Source: CAD feature listing. Evaluate the final solid. Frame: model axes, mm. Round coordinates to 2 decimals unless told otherwise and drop trailing zeros. Order: outer loops, then holes, each group sorted by start corner. A loop starts at its lowest first (then second) coordinate and runs counter-clockwise, first axis right, second up. Notation, with made-up numbers: (32, 41) - (80, 41) arc R11 cw to (80, 46) - close; hole circle Ø1 at (-10.5, 89). An arc over 180 degrees is marked (long way). Return JSON: item names as keys, results as strings. Group by question number.
1) Section D-D, the plane y = 4.5. Give the number of separate pieces and of enclosed holes in the cut face, plus the area to 3 significant figures.
2) Section C-C, the plane y = -3. Return loops of the section in (x, z), plus the area to 3 significant figures.
3) Contact query for a flat-ended pin moving along its axis: P1, Ø3, axis at x = -18.1, y = 3.97, coming from the +Z side. Output: stop coordinate, or through.
4) Ray query, line 1 (Y direction, x = -14.5, z = 0.5); line 2 (X direction, y = 6.5, z = 0.8); line 3 (X direction, y = 4.25, z = 0.65). Return the intervals inside material, ascending. Write a range as from..to.
5) Section A-A, the plane y = 6.5. Return loops of the section in (x, z).
6) Section B-B, the plane x = -1. Return loops of the section in (y, z).
7) Mould query, pull axis X, two halves, no side actions, for faces 1 (the flat face through (-18.079, -3.318, 0.704)), 2 (the cylindrical face through (8.047, 3.919, 0.704)), 3 (the flat face through (-3, 11, 1.4)). Classes: pulls with the +X half, pulls with the -X half, needs draft (parallel to the pull), parting line crosses it, or undercut.
```python
from build123d import *

# Parameters (mm, degrees)
SKETCH4_R           = 1.2500000000000009
SKETCH4_R_2         = 1.2499999999999993
BOSS_EXTRUDE1_DEPTH = 1.4
CHAMFER1_SIZE       = 0.4


with BuildPart() as part:
    # Sketch4 → Boss-Extrude1 (new body)
    # profile 1 of 8: a face of its own
    with BuildSketch(Plane(origin=(-1.7e-16, 0, 1.4000000000000032), x_dir=(-1, 0, -1.2e-16), z_dir=(1.2e-16, 0, -1))):
        Polygon((-7.546190091207485, 10.174212835332735), (-7.046190091207492, 10.174212835332735), (15.853809908792503, 10.174212835332744), (16.35380990879248, 10.174212835332744), (16.35380990879248, 10.674212835332737), (-7.546190091207485, 10.674212835332732), align=None)
    # profile 2 of 8: a face of its own
    with BuildSketch(Plane(origin=(-1.7e-16, 0, 1.4000000000000032), x_dir=(-1, 0, -1.2e-16), z_dir=(1.2e-16, 0, -1))):
        Polygon((-11.686815091207489, 10.17421283533274), (-7.546190091207485, 10.174212835332735), (-7.546190091207485, 10.674212835332732), (16.35380990879248, 10.674212835332737), (16.35380990879248, 10.174212835332744), (20.7538099087925, 10.17421283533274), (15.853809908792503, 12.174212835332744), (-7.046190091207496, 12.174212835332744), (-11.65105221022055, 10.294677276551901), align=None)
    # profile 3 of 8: a face of its own
    with BuildSketch(Plane(origin=(-1.7e-16, 0, 1.4000000000000032), x_dir=(-1, 0, -1.2e-16), z_dir=(1.2e-16, 0, -1))):
        with BuildLine():
            Line((16.35380990879248, 10.174212835332744), (16.353809908792496, -2.225787164667265))
            Line((16.353809908792496, -2.225787164667266), (20.4739831765189, -2.2257871646672647))
            ThreePointArc((20.473983176518885, -2.2257871646672385), (20.614466316717532, -2.0161736201746514), (20.753809908793457, -1.8058008223556463))
            Line((20.753809908792505, -1.805800822355394), (20.7538099087925, 10.17421283533274))
            Line((20.7538099087925, 10.17421283533274), (16.35380990879248, 10.174212835332744))
        make_face()
        with Locations(Location((18.103809908792506, 3.9742128353327333, 0), (0, 0, 180))):
            Circle(SKETCH4_R, mode=Mode.SUBTRACT)
    # profile 4 of 8: a face of its own
    with BuildSketch(Plane(origin=(-1.7e-16, 0, 1.4000000000000032), x_dir=(-1, 0, -1.2e-16), z_dir=(1.2e-16, 0, -1))):
        with BuildLine():
            Line((-7.54619009120748, -2.7257871646672593), (-7.54619009120748, -2.225787164667266))
            Line((-7.54619009120748, -2.225787164667266), (-11.946190091207495, -2.225787164667265))
            Line((-11.946190091207495, -2.225787164667265), (-7.046190091207487, -4.225787164667266))
            Line((-7.046190091207487, -4.225787164667266), (15.853809908792512, -4.225787164667266))
            Line((15.85380990879251, -4.225787164667266), (20.36710720596046, -2.383625002557896))
            ThreePointArc((20.367107205960004, -2.3836250025573023), (20.420626069676963, -2.3047608484368673), (20.473983176518885, -2.2257871646672385))
            Line((20.4739831765189, -2.2257871646672647), (16.353809908792496, -2.225787164667266))
            Line((16.353809908792496, -2.225787164667265), (16.353809908792496, -2.7257871646672562))
            Line((16.353809908792496, -2.725787164667256), (-7.546190091207482, -2.7257871646672593))
        make_face()
    # profile 5 of 8: a face of its own
    with BuildSketch(Plane(origin=(-1.7e-16, 0, 1.4000000000000032), x_dir=(-1, 0, -1.2e-16), z_dir=(1.2e-16, 0, -1))):
        Polygon((15.853809908792512, -2.225787164667266), (-7.046190091207487, -2.225787164667266), (-7.54619009120748, -2.225787164667266), (-7.54619009120748, -2.7257871646672593), (16.353809908792496, -2.725787164667256), (16.353809908792496, -2.225787164667265), align=None)
    # profile 6 of 8: a face of its own
    with BuildSketch(Plane(origin=(-1.7e-16, 0, 1.4000000000000032), x_dir=(-1, 0, -1.2e-16), z_dir=(1.2e-16, 0, -1))):
        Polygon((-11.946190091207495, -2.225787164667265), (-7.54619009120748, -2.225787164667266), (-7.546190091207485, 10.174212835332735), (-11.686815091207489, 10.17421283533274), (-11.946190091207496, 9.300528624806402), align=None)
        with Locations(Location((-9.296190091207496, 3.9742128353327333, 0), (0, 0, 180))):
            Circle(SKETCH4_R_2, mode=Mode.SUBTRACT)
    # profile 7 of 8: a face of its own
    with BuildSketch(Plane(origin=(-1.7e-16, 0, 1.4000000000000032), x_dir=(-1, 0, -1.2e-16), z_dir=(1.2e-16, 0, -1))):
        Polygon((15.853809908792503, 10.174212835332742), (15.85380990879251, -2.225787164667266), (16.353809908792496, -2.225787164667266), (16.35380990879248, 10.174212835332744), align=None)
    # profile 8 of 8: a face of its own
    with BuildSketch(Plane(origin=(-1.7e-16, 0, 1.4000000000000032), x_dir=(-1, 0, -1.2e-16), z_dir=(1.2e-16, 0, -1))):
        Polygon((-7.54619009120748, -2.225787164667266), (-7.046190091207487, -2.225787164667266), (-7.046190091207492, 10.174212835332735), (-7.546190091207485, 10.174212835332735), align=None)
    extrude(amount=BOSS_EXTRUDE1_DEPTH)

    # Chamfer1
    chamfer1_edges = [part.edges().sort_by_distance(p)[0] for p in [
        (8.046190091207496, 3.974212835332733, 1.4000000000000041),
        (-19.353809908792506, 3.974212835332733, 1.4000000000000008),
        (-4.403809908792507, 10.17421283533274, 1.4000000000000028),
        (7.04619009120749, 3.974212835332734, 1.4000000000000041),
        (-4.403809908792514, -2.2257871646672656, 1.4000000000000028),
        (-15.853809908792506, 3.9742128353327377, 1.4000000000000012),
        (11.798621150714023, 9.797602950679153, 1.4000000000000048),
        (9.348621150714022, 11.234445055942324, 1.4000000000000044),
        (-4.403809908792503, 12.174212835332744, 1.4000000000000028),
        (-18.303809908792502, 11.174212835332742, 1.400000000000001),
        (-20.753809908792505, 4.184206006488673, 1.4000000000000008),
        (-20.56153855062731, -2.095435686482624, 1.4000000000000008),
        (-18.110458557376482, -3.3047060836125812, 1.400000000000001),
        (-4.403809908792512, -4.225787164667266, 1.4000000000000028),
        (9.496190091207492, -3.2257871646672656, 1.4000000000000044),
        (11.946190091207495, 3.5373707300695685, 1.4000000000000048),
        (11.798621150714023, 9.797602950679153, 4.78e-15),
        (7.04619009120749, 3.974212835332734, 4.19e-15),
        (-4.40380990879251, -2.2257871646672656, 2.79e-15),
        (-15.853809908792506, 3.9742128353327377, 1.39e-15),
        (8.046190091207496, 3.974212835332733, 4.32e-15),
        (-19.353809908792506, 3.974212835332733, 9.6e-16),
        (9.348621150714022, 11.234445055942324, 4.48e-15),
        (-4.403809908792503, 12.174212835332744, 2.79e-15),
        (-18.303809908792502, 11.174212835332742, 1.09e-15),
        (-20.753809908792505, 4.184206006488673, 7.9e-16),
        (-20.56153855062727, -2.095435686482599, 8.1e-16),
        (-18.110458557376482, -3.3047060836125812, 1.11e-15),
        (-4.403809908792512, -4.225787164667266, 2.79e-15),
        (9.496190091207492, -3.2257871646672656, 4.49e-15),
        (11.946190091207495, 3.5373707300695685, 4.79e-15),
        (-4.403809908792507, 10.17421283533274, 2.79e-15),
    ]]
    chamfer(chamfer1_edges, length=CHAMFER1_SIZE)


solid = part.part
```
Geometry check:
{
 "1": {"separate pieces": "4", "enclosed holes": "0", "area": "6.04 mm2"},
 "2": {"outline": "(-18.86, 0.4) - (-17.8, 0) - (8.99, 0) - (10.05, 0.4) - (10.05, 1) - (8.99, 1.4) - (-17.8, 1.4) - (-18.86, 1) - close", "area": "39.6 mm2"},
 "3": {"P1": "z = 1.26"},
 "4": {"line 1": "-4.23..-2.23, 10.17..12.17", "line 2": "-20.75..-15.85, 7.05..11.95", "line 3": "-20.75..-19.32, -16.88..-15.85, 7.05..8.08, 10.52..11.95"},
 "5": {"outline": "(-20.75, 0.4) - (-20.35, 0) - (-16.25, 0) - (-15.85, 0.4) - (-15.85, 1) - (-16.25, 1.4) - (-20.35, 1.4) - (-20.75, 1) - close; (7.05, 0.4) - (7.45, 0) - (11.55, 0) - (11.95, 0.4) - (11.95, 1) - (11.55, 1.4) - (7.45, 1.4) - (7.05, 1) - close"},
 "6": {"outline": "(-4.23, 0.4) - (-3.83, 0) - (-2.63, 0) - (-2.23, 0.4) - (-2.23, 1) - (-2.63, 1.4) - (-3.83, 1.4) - (-4.23, 1) - close; (10.17, 0.4) - (10.57, 0) - (11.77, 0) - (12.17, 0.4) - (12.17, 1) - (11.77, 1.4) - (10.57, 1.4) - (10.17, 1) - close"},
 "7": {"face 1": "pulls with the -X half", "face 2": "undercut", "face 3": "needs draft"}
}
